```python
from build123d import *

# Parameters (mm, degrees)
SKETCH_R        = 7
SKETCH_R_2      = 1.7
PAD_DEPTH       = 5
SKETCH001_R     = 8.5
SKETCH001_W     = 6.2
SKETCH001_H     = 20
POCKET_DEPTH    = 2.5
FILLET_R        = 4
FILLET001_R     = 4
FILLET002_R     = 4
FILLET003_R     = 4
FILLET004_R     = 4
FILLET005_R     = 4
FILLET006_R     = 1
CHAMFER_SIZE    = 1.5
CHAMFER001_SIZE = 1.5
CHAMFER002_SIZE = 1.5
CHAMFER003_SIZE = 1.5
CHAMFER004_SIZE = 1.5
CHAMFER005_SIZE = 1.5


with BuildPart() as part:
    # Sketch → Pad (new body)
    with BuildSketch(Plane.XY):
        Polygon((-12.5, -12.5), (12.5, -12.5), (12.5, 12.5), (9, 28.5), (-9, 28.5), (-12.5, 12.5), align=None)
        Circle(SKETCH_R, mode=Mode.SUBTRACT)
        with Locations((-8, 8.5)):
            Circle(SKETCH_R_2, mode=Mode.SUBTRACT)
        with Locations((8, 8.5)):
            Circle(SKETCH_R_2, mode=Mode.SUBTRACT)
        with Locations((-8, -8.5)):
            Circle(SKETCH_R_2, mode=Mode.SUBTRACT)
        with Locations((8, -8.5)):
            Circle(SKETCH_R_2, mode=Mode.SUBTRACT)
        with Locations((-6, 23)):
            Circle(SKETCH_R_2, mode=Mode.SUBTRACT)
        with Locations((6, 23)):
            Circle(SKETCH_R_2, mode=Mode.SUBTRACT)
    extrude(amount=PAD_DEPTH)

    # Sketch001 → Pocket (cut)
    with BuildSketch(Plane.XY.offset(5)):
        Circle(SKETCH001_R)
        with Locations((0, 20)):
            Rectangle(SKETCH001_W, SKETCH001_H)
    extrude(amount=-POCKET_DEPTH, mode=Mode.SUBTRACT)

    # Fillet
    fillet_edges = [part.edges().sort_by_distance(p)[0] for p in [
        (-12.5, -12.5, 2.5),
    ]]
    fillet(fillet_edges, radius=FILLET_R)

    # Fillet001
    fillet001_edges = [part.edges().sort_by_distance(p)[0] for p in [
        (12.5, -12.5, 2.5),
    ]]
    fillet(fillet001_edges, radius=FILLET001_R)

    # Fillet002
    fillet002_edges = [part.edges().sort_by_distance(p)[0] for p in [
        (-12.5, 12.5, 2.5),
    ]]
    fillet(fillet002_edges, radius=FILLET002_R)

    # Fillet003
    fillet003_edges = [part.edges().sort_by_distance(p)[0] for p in [
        (12.5, 12.5, 2.5),
    ]]
    fillet(fillet003_edges, radius=FILLET003_R)

    # Fillet004
    fillet004_edges = [part.edges().sort_by_distance(p)[0] for p in [
        (9, 28.5, 2.5),
    ]]
    fillet(fillet004_edges, radius=FILLET004_R)

    # Fillet005
    fillet005_edges = [part.edges().sort_by_distance(p)[0] for p in [
        (-9, 28.5, 2.5),
    ]]
    fillet(fillet005_edges, radius=FILLET005_R)

    # Fillet006
    fillet006_edges = [part.edges().sort_by_distance(p)[0] for p in [
        (0, 28.5, 0),
    ]]
    fillet(fillet006_edges, radius=FILLET006_R)

    # Chamfer
    chamfer_edges = [part.edges().sort_by_distance(p)[0] for p in [
        (-9.7, -8.5, 0),
    ]]
    chamfer(chamfer_edges, length=CHAMFER_SIZE)

    # Chamfer001
    chamfer001_edges = [part.edges().sort_by_distance(p)[0] for p in [
        (-9.7, 8.5, 0),
    ]]
    chamfer(chamfer001_edges, length=CHAMFER001_SIZE)

    # Chamfer002
    chamfer002_edges = [part.edges().sort_by_distance(p)[0] for p in [
        (6.3, -8.5, 0),
    ]]
    chamfer(chamfer002_edges, length=CHAMFER002_SIZE)

    # Chamfer003
    chamfer003_edges = [part.edges().sort_by_distance(p)[0] for p in [
        (6.3, 8.5, 0),
    ]]
    chamfer(chamfer003_edges, length=CHAMFER003_SIZE)

    # Chamfer004
    chamfer004_edges = [part.edges().sort_by_distance(p)[0] for p in [
        (4.3, 23, 0),
    ]]
    chamfer(chamfer004_edges, length=CHAMFER004_SIZE)

    # Chamfer005
    chamfer005_edges = [part.edges().sort_by_distance(p)[0] for p in [
        (-7.7, 23, 0),
    ]]
    chamfer(chamfer005_edges, length=CHAMFER005_SIZE)


solid = part.part
```
Here's how the part is built. I have some questions about the finished solid (model axes, mm). A direction names the side the tool comes from. Round coordinates to 2 decimals unless told otherwise and drop trailing zeros. Order: outer loops, then holes, each group sorted by start corner. A loop starts at its lowest first (then second) coordinate and runs counter-clockwise, first axis right, second up. Notation, with made-up numbers: M 28.25,16.25 L 70.25,16.25 A8 ccw 70.25,26.25 Z; hole C 76.5,73.5 d11. An arc over 180 degrees is marked long. Use CSV: the item, a comma, the result in double quotes.
1) I want a section at C-C (x = 1.5). List the corners of the cut face in (y, z) for me.
Taken from the geometry:
outline,"M -12.5,1 A1 ccw -11.5,0 L -6.84,0 L -6.84,2.5 L -8.37,2.5 L -8.37,5 L -12.5,5 Z; M 6.84,0 L 27.5,0 A1 ccw 28.5,1 L 28.5,2.5 L 10,2.5 L 10,5 L 8.37,5 L 8.37,2.5 L 6.84,2.5 Z"
2) I want a section at B-B (z = 4.3). List the corners of the cut face in (x, y) for me, then the cut area to 3 significant figures.
Taken from the geometry:
outline,"M -12.5,-8.5 A4 ccw -8.5,-12.5 L 8.5,-12.5 A4 ccw 12.5,-8.5 L 12.5,12.07 A4 ccw 12.41,12.92 L 9.69,25.35 A4 ccw 5.78,28.5 L 3.1,28.5 L 3.1,10 L -3.1,10 L -3.1,28.5 L -5.78,28.5 A4 ccw -9.69,25.35 L -12.41,12.92 A4 ccw -12.5,12.07 Z; hole C -8,-8.5 d3.4; hole C -8,8.5 d3.4; hole C 0,0 d17; hole C -6,23 d3.4; hole C 6,23 d3.4; hole C 8,-8.5 d3.4; hole C 8,8.5 d3.4"
area,"562 mm^2"
3) I'm going to push flat-ended pins straight in: P1, Ø5, axis at x = -3.5, y = 2.5, coming from the +Z side; P2, Ø2, axis at y = 21, z = 3.5, coming from the +X side; P3, Ø5, axis at x = 0.5, y = 15.5, coming from the +Z side; P4, Ø2, axis at y = 15.5, z = 3, coming from the -X side. Where does each tip first touch, or does it pass through?
Taken from the geometry:
P1,"through"
P2,"x = 10.86"
P3,"z = 2.5"
P4,"x = -12.06"
4) I want a section at D-D (y = 22). Count the separate pieces of the cut face and the enclosed holes in it, then the cut area to 3 significant figures.
Taken from the geometry:
separate pieces,"3"
enclosed holes,"0"
area,"55.7 mm^2"
5) I need wall thicknesses on line 1 along Y through (x, z) = (6, 0.85); line 2 along Y through (x, z) = (0, 3.65); line 3 along X through (y, z) = (23, 2.9). Which ranges of each line are inside material? Lowest first, please. Write a range as [from, to].
Taken from the geometry:
line 1,"[-12.49, -9.73], [-7.27, -3.61], [3.61, 7.27], [9.73, 20.65], [25.35, 28.48]"
line 2,"[-12.5, -8.5], [8.5, 10]"
line 3,"[-10.2, -7.7], [-4.3, -3.1], [3.1, 4.3], [7.7, 10.2]"
6) If we mould it in two halves opening along X, with no side actions, what happens to faces 4 (the cylindrical face through (-8.26, 27.64, 3.03)), 5 (the cylindrical face through (11.297, -11.359, 3.028)), 6 (the cylindrical face through (7.63, 6.84, 3.23))? For each: pulls with the +X half, pulls with the -X half, needs draft (parallel to the pull), parting line crosses it, or undercut.
Taken from the geometry:
face 4,"pulls with the -X half"
face 5,"pulls with the +X half"
face 6,"undercut"
7) On a 3-axis mill with a long thin cutter (end or side, diameter ignored), from which of +Z, -Z, +X, -X, +Y, -Y can I reach the whole of each face in a straight line? I mean faces 1 (the cylindrical face through (4.57, 7.167, 3.768)), 2 (the cylindrical face through (-12.477, 12.492, 3.028)), 3 (the flat face through (0, 10, 4)). Say none if no direction works.
Taken from the geometry:
face 1,"+Z"
face 2,"+Z, -Z, -X, +Y"
face 3,"+Z, +Y"
8) I want a section at A-A (y = 0). List the corners of the cut face in (x, z) for me, then the cut area to 3 significant figures.
Taken from the geometry:
outline,"M -12.5,1 A1 ccw -11.5,0 L -7,0 L -7,2.5 L -8.5,2.5 L -8.5,5 L -12.5,5 Z; M 7,0 L 11.5,0 A1 ccw 12.5,1 L 12.5,5 L 8.5,5 L 8.5,2.5 L 7,2.5 Z"
area,"47.1 mm^2"
